The drawing under review shows one solid part. Ordinate dimensions are in mm from its lowest x, y, z. Coordinates: 2 decimals unless noted, no trailing zeros. Write each loop counter-clockwise with the first axis right and the second up, starting at its lowest first coordinate (ties: lowest second). Pieces come first, ordered by that corner, then holes.
1) Add section B-B, the plane y = 37. State the section outline as (x, z) points.
2) Add section A-A, the plane z = 4.75. State the section outline as (x, y) points, then the cut area to 3 significant figures.
3) Mouldability with a two-part tool opening along X and no side actions: class the marked faces 1, 2 and 3 as released by +X, released by -X, zero draft, split by the parting line, or undercut.
4) Add section D-D, the plane z = 9.25. State the section outline as (x, y) points.
5) Add section C-C, the plane x = 3. State the section outline as (y, z) points.
6) For line 1 (X direction, y = 2, z = 7); line 2 (Y direction, x = 3, z = 12.75); line 3 (X direction, y = 37, z = 16.25), list the stretches that pass through material, from the lowest coordinate up.
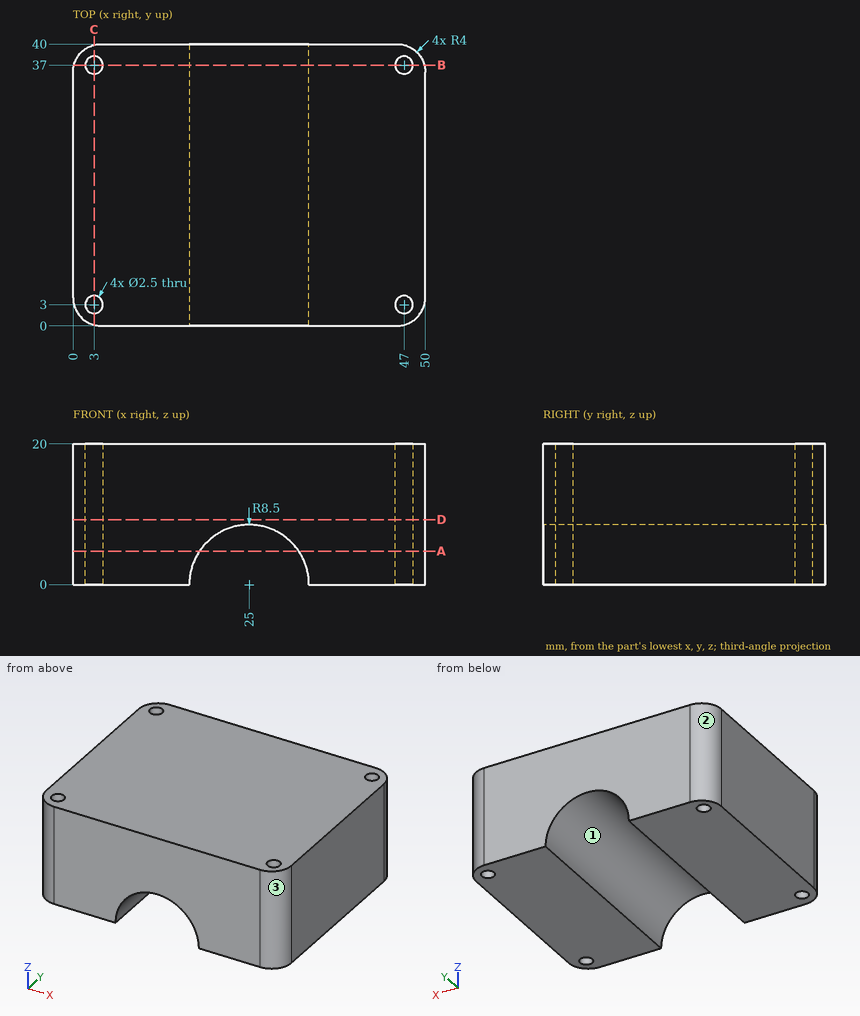
Geometry results:
1. outline: (0.13, 0) - (1.75, 0) - (1.75, 20) - (0.13, 20) - close; (4.25, 0) - (16.5, 0) arc R8.5 cw to (33.5, 0) - (45.75, 0) - (45.75, 20) - (4.25, 20) - close; (48.25, 0) - (49.87, 0) - (49.87, 20) - (48.25, 20) - close
2. outline: (0, 4) arc R4 ccw to (4, 0) - (17.95, 0) - (17.95, 40) - (4, 40) arc R4 ccw to (0, 36) - close; (32.05, 0) - (46, 0) arc R4 ccw to (50, 4) - (50, 36) arc R4 ccw to (46, 40) - (32.05, 40) - close; hole circle Ø2.5 at (3, 3); hole circle Ø2.5 at (3, 37); hole circle Ø2.5 at (47, 3); hole circle Ø2.5 at (47, 37)
2. area: 1,400 mm2
3. face 1: undercut
3. face 2: released by -X
3. face 3: released by +X
4. outline: (0, 4) arc R4 ccw to (4, 0) - (46, 0) arc R4 ccw to (50, 4) - (50, 36) arc R4 ccw to (46, 40) - (4, 40) arc R4 ccw to (0, 36) - close; hole circle Ø2.5 at (3, 3); hole circle Ø2.5 at (3, 37); hole circle Ø2.5 at (47, 3); hole circle Ø2.5 at (47, 37)
5. outline: (0.13, 0) - (1.75, 0) - (1.75, 20) - (0.13, 20) - close; (4.25, 0) - (35.75, 0) - (35.75, 20) - (4.25, 20) - close; (38.25, 0) - (39.87, 0) - (39.87, 20) - (38.25, 20) - close
6. line 1: x = 0.54 to 2.25, 3.75 to 20.18, 29.82 to 46.25, 47.75 to 49.46
6. line 2: y = 0.13 to 1.75, 4.25 to 35.75, 38.25 to 39.87
6. line 3: x = 0.13 to 1.75, 4.25 to 45.75, 48.25 to 49.87
